The model under review builds one solid part; all positions refer to its coordinate system, in mm. Give positions to 0.01 mm unless a question says otherwise; leave off trailing zeros. Loops run counter-clockwise (first coordinate to the right, second up) from the corner with the lowest first, then second, coordinate; pieces in that order, holes last. Notation, with made-up numbers: M 79,-19.75 L 118,-19.75 A33 ccw 118,13.25 Z; hole C 71.5,-35.5 d6. An arc over 180 degrees is marked long. Return JSON: item names as keys, results as strings. Group by question number.
```python
from build123d import *

# Parameters (mm, degrees)
SKETCH_W     = 40
SKETCH_H     = 35
PAD_DEPTH    = 15
SKETCH001_R  = 2.25
HOLE_DEPTH   = 25
CHAMFER_SIZE = 2


with BuildPart() as part:
    # Sketch → Pad (new body)
    with BuildSketch(Plane.XY):
        Rectangle(SKETCH_W, SKETCH_H)
    extrude(amount=-PAD_DEPTH)

    # Sketch001 → Hole (cut)
    with BuildSketch(Plane.XY):
        with Locations((-13, 13)):
            Circle(SKETCH001_R)
        with Locations((13, 13)):
            Circle(SKETCH001_R)
        with Locations((13, -13)):
            Circle(SKETCH001_R)
        with Locations((-13, -13)):
            Circle(SKETCH001_R)
    extrude(amount=-HOLE_DEPTH, mode=Mode.SUBTRACT)

    # Chamfer
    chamfer_edges = [part.edges().sort_by_distance(p)[0] for p in [
        (-20, -17.5, -7.5),
        (20, -17.5, -7.5),
        (-20, 17.5, -7.5),
        (20, 17.5, -7.5),
    ]]
    chamfer(chamfer_edges, length=CHAMFER_SIZE)


solid = part.part
```
(1) For probe 1 along Y at (x, z) = (13, -3); probe 2 along X at (y, z) = (14.5, -8); probe 3 along Y at (x, z) = (15, -11.5), list the stretches that pass through material, from the lowest coordinate up.
(2) Mouldability with a two-part tool opening along Y and no side actions: class faces 1 (the cylindrical face through (-14.66, -11.48, -7.4)), 2 (the flat face through (0, 0, 0)), 3 (the cylindrical face through (-14.66, 14.52, -7.4)), 4 (the flat face through (-19, 16.5, -7.4)) as released by +Y, released by -Y, zero draft, split by the parting line, or undercut.
(3) Add section A-A (y = 13). Write out the cut boundary in (x, z).
(4) Add section C-C (z = -10). Write out the cut boundary in (x, y).
(5) Add section B-B (x = -13). Write out the cut boundary in (y, z).
Verdict:
{
 "1": {"probe 1": "y = -17.5 to -15.25, -10.75 to 10.75, 15.25 to 17.5", "probe 2": "x = -20 to -14.68, -11.32 to 11.32, 14.68 to 20", "probe 3": "y = -17.5 to -14.03, -11.97 to 11.97, 14.03 to 17.5"},
 "2": {"face 1": "undercut", "face 2": "zero draft", "face 3": "undercut", "face 4": "released by +Y"},
 "3": {"outline": "M -20,-15 L -15.25,-15 L -15.25,0 L -20,0 Z; M -10.75,-15 L 10.75,-15 L 10.75,0 L -10.75,0 Z; M 15.25,-15 L 20,-15 L 20,0 L 15.25,0 Z"},
 "4": {"outline": "M -20,-15.5 L -18,-17.5 L 18,-17.5 L 20,-15.5 L 20,15.5 L 18,17.5 L -18,17.5 L -20,15.5 Z; hole C -13,-13 d4.5; hole C -13,13 d4.5; hole C 13,-13 d4.5; hole C 13,13 d4.5"},
 "5": {"outline": "M -17.5,-15 L -15.25,-15 L -15.25,0 L -17.5,0 Z; M -10.75,-15 L 10.75,-15 L 10.75,0 L -10.75,0 Z; M 15.25,-15 L 17.5,-15 L 17.5,0 L 15.25,0 Z"}
}
